Geometry check sheet. Reference: the model listing, model coordinates, mm. Round coordinates to 2 decimals unless told otherwise and drop trailing zeros. Loops run counter-clockwise (first coordinate to the right, second up) from the corner with the lowest first, then second, coordinate; pieces in that order, holes last. Notation, with made-up numbers: (-34.5, -34) -> (20.5, -34) arc R6 cw to (20.5, -26) -> close; hole circle Ø11 at (18.5, -1). An arc over 180 degrees is marked (long way). Use a Markdown table: item, result. Add a question column.
Q1. Gauge pin test, flat ends, axial feed: P1, Ø5, axis at x = -2.5, z = 119, coming from the +Y side; P2, Ø5, axis at y = 5, z = 44.5, coming from the +X side; P3, Ø1.5, axis at x = 1.5, y = 6, coming from the +Z side. Record the tip position at first contact, or that the pin passes through.
Q2. Sectioned sample at A-A, the plane z = 29.5. Enter the section's corners in (x, y).
Q3. Material ranges on L1, parallel to Z at x = 0, y = -8; L2, parallel to Z at x = -4, y = 7.5; L3, parallel to Y at x = -0.5, z = 30, recorded low to high.
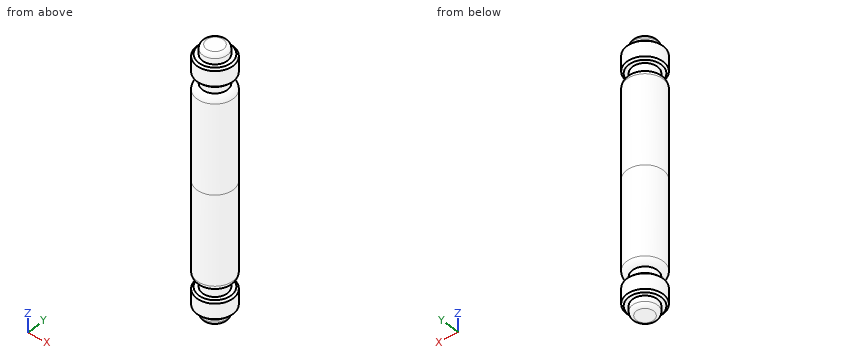
```python
from build123d import *

# Parameters (mm, degrees)
F4_SIZE = 1


with BuildPart() as f1:
    # F0 (on Front) → F1 (revolve)
    with BuildSketch(Plane.XZ):
        with BuildLine():
            Line((0, 70), (0, 0))
            Line((0, 0), (4.5, 0))
            ThreePointArc((4.5, 0), (5.9142135624, 0.5857864376), (6.5, 2))
            Line((6.5, 2), (6.5, 5))
            Line((6.5, 5), (9.5, 5))
            Line((9.5, 5), (9.5, 15))
            Line((9.5, 15), (6.5, 15))
            Line((6.5, 15), (6.5, 20))
            ThreePointArc((6.5, 20), (8.6213203436, 20.8786796564), (9.5, 23))
            Line((9.5, 23), (9.5, 70))
            Line((9.5, 70), (0, 70))
        make_face()
    revolve(axis=Axis((0, 0, 35), (0, 0, 1)))

    # F3: F1 across plane


with BuildPart() as f1_1:
    add(f1.part)
    add(f1.part.mirror(Plane.XY.offset(70)))

    # F4
    f4_edges = [f1_1.edges().sort_by_distance(p)[0] for p in [
        (-9.5, 0, 135),
        (-9.5, 0, 125),
        (9.5, 0, 130),
        (-9.5, 0, 5),
        (-9.5, 0, 15),
        (9.5, 0, 10),
    ]]
    chamfer(f4_edges, length=F4_SIZE)


solid = f1_1.part
```
Values:
| question | item | result |
|---|---|---|
| 1 | P1 | y = 9.46 |
| 1 | P2 | x = 9.17 |
| 1 | P3 | z = 139.77 |
| 2 | outline | circle Ø19 at (0, 0) |
| 3 | L1 | 5 to 15, 20.4 to 119.6, 125 to 135 |
| 3 | L2 | 5 to 15, 20.76 to 119.24, 125 to 135 |
| 3 | L3 | -9.49 to 9.49 |
